Autodesk Inventor part; units mm, degrees
ref_plane "YZ Plane" through (0, 0, 0) normal (1, 0, 0) x (0, 1, 0)
ref_plane "XZ Plane" through (0, 0, 0) normal (0, 1, 0) x (-1, 0, 0)
ref_plane "XY Plane" through (0, 0, 0) normal (0, 0, 1) x (1, 0, 0)
sketch "Sketch1" plane through (0, 0, 0) normal (0, 0, 1) x (1, 0, 0)
  line L0 (0, 0) -> (1, 0)
  line L1 (1, 0) -> (1, 7.5)
  line L2 (1, 7.5) -> (0, 7.5)
  line L3 (0, 7.5) -> (0, 0)
  dimension "d0" = 1
  dimension "d1" = 7.5
extrude "Extrusion1" add sketch "Sketch1" along normal blind 0.5
sketch "Sketch2" plane through (0, 0, 0) normal (-1, 0, 0) x (0, 0, 1)
  point P0 (0, 0)
sketch "Sketch3" plane through (0, 0, 0) normal (0, 1, 0) x (-1, 0, 0)
  line L0 (0, 0) -> (-1, 0)
  line L1 (0, 0) -> (-1, 0)
  line L2 (-1, 0) -> (-1, 7.5)
  line L3 (-1, 7.5) -> (0, 7.5)
  line L4 (0, 7.5) -> (0, 0)
  dimension "d4" = 1
  dimension "d5" = 7.5
extrude "Extrusion2" add sketch "Sketch3" along normal blind 0.5
sketch "Sketch4" plane through (0, 0, 0.5) normal (0, 0, 1) x (1, 0, 0)
  line L0 (0, 7.9375) -> (0, 6.4375)
  line L1 (0, 6.4375) -> (0.5, 6.4375)
  circle A0 centre (0.5, 6.4375) radius 0.15
  point P0 (0, 0)
  dimension "d8" = 1.5
  dimension "d9" = 0.5
  dimension "d10" = 0.3
extrude "Extrusion3" cut sketch "Sketch4" against normal through all
sketch "Sketch5" plane through (0, 0.5, 0) normal (0, 1, 0) x (1, 0, 0)
  line L0 (0, 0) -> (0, -7.5)
  line L1 (0, -7.5) -> (0, -6)
  line L2 (0, -6) -> (0.5, -6)
  line L3 (1, 0) -> (1, -7.5)
  circle A0 centre (0.5, -6) radius 0.15
  dimension "d13" = 1.5
  dimension "d14" = 0.5
  dimension "d15" = 0.3
extrude "Extrusion4" cut sketch "Sketch5" against normal through all
properties part number "CLAMP"
Build history of the part. All positions in model axes, mm. A direction names the side the tool comes from. Coordinates: 2 decimals unless noted, no trailing zeros. Order: outer loops, then holes, each group sorted by start corner. A loop starts at its lowest first (then second) coordinate and runs counter-clockwise, first axis right, second up. Notation, with made-up numbers: (-4, 23.25) -> (24, 23.25) arc R33 ccw to (24, 62.25) -> close; hole circle Ø1 at (-3, 56). An arc over 180 degrees is marked (long way). Answer in a Markdown table with one row per item. Add a question column.
Q1. Band-saw the part on B-B, the plane x = 0.5. List the corners of the cut face in (y, z).
Q2. Band-saw the part on A-A, the plane z = 6. List the corners of the cut face in (x, y).
Q3. Which spindle directions (+Z, -Z, +X, -X, +Y, -Y) get a long thin tool onto all of the face, cutting with end or side? Do faces 1 (the face through (0.5, 3.8, 0)), 2 (the face through (0.5, 0.5, 4)). Say none if no direction does.
Q4. Band-saw the part on C-C, the plane y = 7.25. List the corners of the cut face in (x, z), then the cut area to 3 significant figures.
Q5. Drop flat-ended pins along their axis: pin 1 (0.5 mm diameter, centred on x = 0.5, z = 3, fed in from +Y); pin 2 (2 mm diameter, centred on y = 5, z = 3, fed in from -X); pin 3 (4 mm diameter, centred on y = 1, z = 2.5, fed in from -X). Give the stop position or say it passes through.
Q6. Wall check: line 1 along Y through (x, z) = (0.25, 3.75); line 2 along Y through (x, z) = (0.5, 0.15). Give the ranges that are in metal, low to high. Write a range as [from, to].
Answers follow:
| question | item | result |
|---|---|---|
| 1 | outline | (0, 0) -> (6.29, 0) -> (6.29, 0.5) -> (0.5, 0.5) -> (0.5, 5.85) -> (0, 5.85) -> close; (0, 6.15) -> (0.5, 6.15) -> (0.5, 7.5) -> (0, 7.5) -> close; (6.59, 0) -> (7.5, 0) -> (7.5, 0.5) -> (6.59, 0.5) -> close |
| 2 | outline | (0, 0) -> (0.35, 0) -> (0.35, 0.5) -> (0, 0.5) -> close; (0.65, 0) -> (1, 0) -> (1, 0.5) -> (0.65, 0.5) -> close |
| 3 | face 1 | -Z, +X, -X, +Y, -Y |
| 3 | face 2 | +Z, +X, -X, +Y |
| 4 | outline | (0, 0) -> (1, 0) -> (1, 0.5) -> (0, 0.5) -> close |
| 4 | area | 0.500 mm^2 |
| 5 | pin 1 | y = 0.5 |
| 5 | pin 2 | through |
| 5 | pin 3 | x = 0 |
| 6 | line 1 | [0, 0.5] |
| 6 | line 2 | [0, 6.29], [6.59, 7.5] |
